The listing builds one solid part. Answer for the finished solid, in the listing's coordinates (mm). Face numbers are marked on the shaded views. A direction names the side the tool comes from. Give positions to 0.01 mm unless a question says otherwise; leave off trailing zeros. Loops run counter-clockwise (first coordinate to the right, second up) from the corner with the lowest first, then second, coordinate; pieces in that order, holes last. Notation, with made-up numbers: (9, -32) - (16, -32) arc R11 ccw to (16, -20) - close; hole circle Ø4 at (46.5, -32.75). An arc over 180 degrees is marked (long way). Answer as CSV lines item,"result". Start each with the question number.
1) A cutting plane is placed at A-A (y = -51). Determine the outline of the cut face in (x, z), and give its area (3 significant figures).
2) For the marked faces 1 and 2, determine the directions among +Z, -Z, +X, -X, +Y, -Y from which every point of the face is accessible in a straight line to the end or side of a thin tool.
3) Flat-ended cylindrical pins translate along their axes: pin 1 (6 mm diameter, centred on x = 79, z = -20.5, fed in from +Y); pin 2 (5 mm diameter, centred on y = -50.5, z = -9.5, fed in from +X); pin 3 (10 mm diameter, centred on y = -46, z = -9.5, fed in from +X). Find the tip coordinate at first contact, or state that the pin passes through.
4) Find the intervals of material crossed by line 1 along Y through (x, z) = (72, -6); line 2 along Y through (x, z) = (58, -9); line 3 along Y through (x, z) = (70.5, -20), in increasing order.
5) A cutting plane is placed at B-B (y = -8). Determine the outline of the cut face in (x, z), and give its area (3 significant figures).
6) For a pull along Y with two mould halves and no side action, classify the marked faces 3, 4 and 5 as pulls with the +Y half, pulls with the -Y half, needs draft (parallel to the pull), parting line crosses it, or undercut.
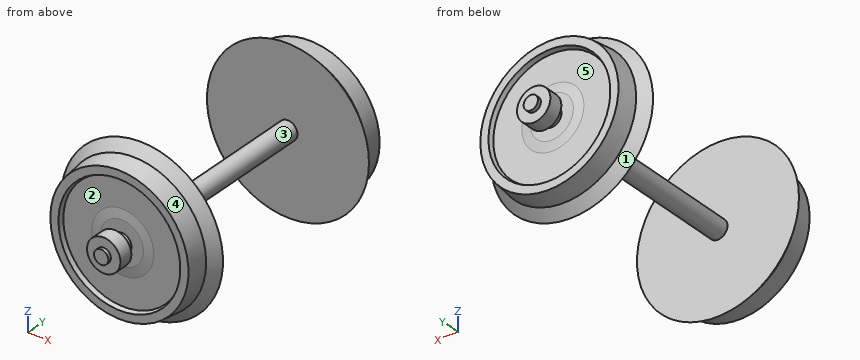
```python
from build123d import *

# Parameters (mm, degrees)
CYLINDER032_R             = 2
CYLINDER032_DEPTH         = 10
CUT021_PLACEMENT_ANGLE    = 180
CYLINDER034_R             = 1.5
CYLINDER034_DEPTH         = 3
CYLINDER033_R             = 3.5
CYLINDER033_DEPTH         = 3
CUT022_PLACEMENT_ANGLE    = 90
CYLINDER030_R             = 1.5
CYLINDER030_DEPTH         = 3
CYLINDER029_R             = 3.5
CYLINDER029_DEPTH         = 3
CUT019_PLACEMENT_ANGLE    = 90
CYLINDER036_R             = 1.5
CYLINDER036_DEPTH         = 62.5
CYLINDER035_R             = 2
CYLINDER035_DEPTH         = 55
FUSION012_PLACEMENT_ANGLE = 90
CYLINDER031_R             = 2
CYLINDER031_DEPTH         = 10


with BuildPart() as cylinder032:
    # Cylinder032 → Cylinder032 (new body)
    with BuildSketch(Plane.XZ.offset(-8)):
        Circle(CYLINDER032_R)
    extrude(amount=CYLINDER032_DEPTH)


with BuildPart() as rad004:
    # Sketch005 → Revolve004 (revolve)
    with BuildSketch(Plane.XY):
        Polygon((0, 0), (17, 0), (15, 2), (14.5, 6.2), (12.8, 6.2), (12.5, 5.25), (6.5, 5.25), (4.5, 5.5), (0, 5.5), align=None)
    revolve(axis=Axis((0, 0, 0), (0, -1, 0)))

    # Cut021: cut Cylinder032
    add(cylinder032.part, mode=Mode.SUBTRACT)


with BuildPart() as rad004_1:
    # Cut021 placement: moved
    add(rad004.part.moved(Location((0, -40, 0))).rotate(Axis((0, -40, 0), (0, 0, 1)), CUT021_PLACEMENT_ANGLE))


with BuildPart() as cylinder034:
    # Cylinder034 → Cylinder034 (new body)
    with BuildSketch(Plane.XY):
        Circle(CYLINDER034_R)
    extrude(amount=CYLINDER034_DEPTH)


with BuildPart() as kugellager004:
    # Cylinder033 → Cylinder033 (new body)
    with BuildSketch(Plane.XY):
        Circle(CYLINDER033_R)
    extrude(amount=CYLINDER033_DEPTH)

    # Cut022: cut Cylinder034
    add(cylinder034.part, mode=Mode.SUBTRACT)


with BuildPart() as kugellager004_1:
    # Cut022 placement: moved
    add(kugellager004.part.moved(Location((0, -47.5, 0))).rotate(Axis((0, -47.5, 0), (1, 0, 0)), CUT022_PLACEMENT_ANGLE))


with BuildPart() as cylinder030:
    # Cylinder030 → Cylinder030 (new body)
    with BuildSketch(Plane.XY):
        Circle(CYLINDER030_R)
    extrude(amount=CYLINDER030_DEPTH)


with BuildPart() as kugellager003:
    # Cylinder029 → Cylinder029 (new body)
    with BuildSketch(Plane.XY):
        Circle(CYLINDER029_R)
    extrude(amount=CYLINDER029_DEPTH)

    # Cut019: cut Cylinder030
    add(cylinder030.part, mode=Mode.SUBTRACT)


with BuildPart() as kugellager003_1:
    # Cut019 placement: moved
    add(kugellager003.part.moved(Location((0, 10.5, 0))).rotate(Axis((0, 10.5, 0), (1, 0, 0)), CUT019_PLACEMENT_ANGLE))


with BuildPart() as cylinder036:
    # Cylinder036 → Cylinder036 (new body)
    with BuildSketch(Plane.XY):
        Circle(CYLINDER036_R)
    extrude(amount=CYLINDER036_DEPTH)


with BuildPart() as achse003:
    # Cylinder035 → Cylinder035 (new body)
    with BuildSketch(Plane.XY.offset(3.75)):
        Circle(CYLINDER035_R)
    extrude(amount=CYLINDER035_DEPTH)

    # Fusion012: union Cylinder036
    add(cylinder036.part)


with BuildPart() as achse003_1:
    # Fusion012 placement: moved
    add(achse003.part.moved(Location((0, 11.3, 0))).rotate(Axis((0, 11.3, 0), (1, 0, 0)), FUSION012_PLACEMENT_ANGLE))


with BuildPart() as cylinder031:
    # Cylinder031 → Cylinder031 (new body)
    with BuildSketch(Plane.XZ.offset(-8)):
        Circle(CYLINDER031_R)
    extrude(amount=CYLINDER031_DEPTH)


with BuildPart() as obj1:
    # Sketch005 → Revolve003 (revolve)
    with BuildSketch(Plane.XY):
        Polygon((0, 0), (17, 0), (15, 2), (14.5, 6.2), (12.8, 6.2), (12.5, 5.25), (6.5, 5.25), (4.5, 5.5), (0, 5.5), align=None)
    revolve(axis=Axis((0, 0, 0), (0, -1, 0)))

    # Cut020: cut Cylinder031
    add(cylinder031.part, mode=Mode.SUBTRACT)

    # Fusion013: union Rad004, Kugellager004, Kugellager003, Achse003
    add(rad004_1.part)
    add(kugellager004_1.part)
    add(kugellager003_1.part)
    add(achse003_1.part)


with BuildPart() as obj1_1:
    # Fusion013 placement: moved
    add(obj1.part.moved(Location((70.08, -11.75, -7))))


solid = obj1_1.part
```
Ans:
1,outline,"circle Ø4 at (70.08, -7)"
1,area,"12.6 mm2"
2,face 1,"+Y"
2,face 2,"-Y"
3,pin 1,"y = -5.55"
3,pin 2,"x = 87.08"
3,pin 3,"x = 72.08"
4,line 1,"-62.25 to -59.25, -57.25 to -51.75, -11.75 to -6.25, -4.25 to -1.25"
4,line 2,"-57 to -51.75, -11.75 to -6.5"
4,line 3,"-57.95 to -51.75, -11.75 to -5.55"
5,outline,"circle Ø29.58 at (70.08, -7)"
5,area,"687 mm2"
6,face 3,"undercut"
6,face 4,"pulls with the -Y half"
6,face 5,"pulls with the +Y half"
